from build123d import *

# Parameters (mm, degrees)
CORTAR_EXTRUIR1_DEPTH      = 12.5875
CORTAR_EXTRUIR1_DEPTH_BACK = 12.5875
CORTAR_EXTRUIR2_DEPTH      = 12.5875001
CORTAR_EXTRUIR2_DEPTH_BACK = 12.5875001
CORTAR_EXTRUIR3_DEPTH      = 12.5875001
CORTAR_EXTRUIR3_DEPTH_BACK = 12.5875001


with BuildPart() as part:
    # Croquis1 → Revolución1 (revolve)
    with BuildSketch(Plane.XY):
        Polygon((-61.538063792, 11.5875), (-19.948063792, 11.5875), (-19.948063792, 8.4125), (-17.448063792, 8.4125), (-17.448063792, 2.38125), (0, 2.38125), (0, 1.5875), (-17.448063792, 1.5875), (-21.538063792, 1.5875), (-21.538063792, 10), (-61.538063792, 10), align=None)
    revolve(axis=Axis((0, 0, 0), (-1, 0, 0)))

    # Croquis2 → Cortar-Extruir1 (cut, two sides)
    with BuildSketch(Plane.XY) as cortar_extruir1_sk:
        with BuildLine():
            Line((-40, 2.5), (-30, 2.5))
            ThreePointArc((-30, 2.5), (-27.5, 0), (-30, -2.5))
            Line((-30, -2.5), (-40, -2.5))
            ThreePointArc((-40, -2.5), (-42.5, 0), (-40, 2.5))
        make_face()
    extrude(amount=CORTAR_EXTRUIR1_DEPTH, mode=Mode.SUBTRACT)
    extrude(cortar_extruir1_sk.sketch, amount=-CORTAR_EXTRUIR1_DEPTH_BACK, mode=Mode.SUBTRACT)

    # Croquis3 → Cortar-Extruir2 (cut, two sides)
    with BuildSketch(Plane(origin=(0, 0, 0), x_dir=(1, 0, 0), z_dir=(0, 1, 0))) as cortar_extruir2_sk:
        with BuildLine():
            Line((-40, 2.5), (-30, 2.5))
            ThreePointArc((-30, 2.5), (-27.5, 0), (-30, -2.5))
            Line((-30, -2.5), (-40, -2.5))
            ThreePointArc((-40, -2.5), (-42.5, 0), (-40, 2.5))
        make_face()
    extrude(amount=CORTAR_EXTRUIR2_DEPTH, mode=Mode.SUBTRACT)
    extrude(cortar_extruir2_sk.sketch, amount=-CORTAR_EXTRUIR2_DEPTH_BACK, mode=Mode.SUBTRACT)

    # Croquis4 → Cortar-Extruir3 (cut, two sides)
    with BuildSketch(Plane.XY) as cortar_extruir3_sk:
        Polygon((0, 2.38125), (-0.839757246, -2.38125), (0, -2.38125), align=None)
    extrude(amount=CORTAR_EXTRUIR3_DEPTH, mode=Mode.SUBTRACT)
    extrude(cortar_extruir3_sk.sketch, amount=-CORTAR_EXTRUIR3_DEPTH_BACK, mode=Mode.SUBTRACT)


solid = part.part
The model under review builds one solid part; all positions refer to its coordinate system, in mm. A direction names the side the tool comes from. Coordinates: 2 decimals unless noted, no trailing zeros. Write each loop counter-clockwise with the first axis right and the second up, starting at its lowest first coordinate (ties: lowest second). Pieces come first, ordered by that corner, then holes. Notation, with made-up numbers: M 73.25,5.25 L 112.25,5.25 A8 ccw 112.25,19.25 Z; hole C -28.5,11 d2. An arc over 180 degrees is marked long. Put each result on its own line as item: value.
1) Add section C-C on y = 0. Give the boundary of the cut face in (x, z).
Computed:
outline: M -61.54,-11.59 L -42.5,-11.59 L -42.5,-10 L -61.54,-10 Z; M -61.54,10 L -42.5,10 L -42.5,11.59 L -61.54,11.59 Z; M -27.5,-11.59 L -19.95,-11.59 L -19.95,-8.41 L -17.45,-8.41 L -17.45,-2.38 L -0.42,-2.38 L -0.42,-1.59 L -21.54,-1.59 L -21.54,-10 L -27.5,-10 Z; M -27.5,10 L -21.54,10 L -21.54,1.59 L -0.42,1.59 L -0.42,2.38 L -17.45,2.38 L -17.45,8.41 L -19.95,8.41 L -19.95,11.59 L -27.5,11.59 Z
2) Add section D-D on x = -5.5. Give the boundary of the cut face in (y, z) (1 decimal), then the cut area to 3 significant figures.
Computed:
outline: C 0,0 d4.8; hole C 0,0 d3.2
area: 9.90 mm2
3) Add section A-A on x = -35.5. Give the boundary of the cut face in (y, z) (1 decimal), then the cut area to 3 significant figures.
Computed:
outline: M -11.3,-2.5 A11.6 ccw -2.5,-11.3 L -2.5,-9.7 A10 cw -9.7,-2.5 Z; M -11.3,2.5 L -9.7,2.5 A10 cw -2.5,9.7 L -2.5,11.3 A11.6 ccw Z; M 2.5,-11.3 A11.6 ccw 11.3,-2.5 L 9.7,-2.5 A10 cw 2.5,-9.7 Z; M 2.5,9.7 A10 cw 9.7,2.5 L 11.3,2.5 A11.6 ccw 2.5,11.3 Z
area: 75.6 mm2
4) Add section B-B on z = -0.75. Give the boundary of the cut face in (x, y).
Computed:
outline: M -61.54,-11.56 L -42.38,-11.56 L -42.38,-9.97 L -61.54,-9.97 Z; M -61.54,9.97 L -42.38,9.97 L -42.38,11.56 L -61.54,11.56 Z; M -27.62,-11.56 L -19.95,-11.56 L -19.95,-8.38 L -17.45,-8.38 L -17.45,-2.26 L -0.82,-2.26 L -0.67,-1.4 L -21.54,-1.4 L -21.54,-9.97 L -27.62,-9.97 Z; M -27.62,9.97 L -21.54,9.97 L -21.54,1.4 L -0.17,1.4 L -0.02,2.26 L -17.45,2.26 L -17.45,8.38 L -19.95,8.38 L -19.95,11.56 L -27.62,11.56 Z
5) For faces 4 (the cylindrical face through (-27.5, -10.6, -0.1)), 5 (the flat face through (-19.948, -6.1, -6.1)), 6 (the cylindrical face through (-42.5, -0.1, 10.6)), 7 (the cylindrical face through (-40.45, 5.35, 10.28)), list the 3-axis set-ups (+Z, -Z, +X, -X, +Y, -Y) from which the entire face can be reached by the end or side of a thin tool; tool diameter is ignored.
Computed:
face 4: +Y, -Y
face 5: +X
face 6: +Z, -Z
face 7: +X, -X
6) Draft analysis for pull direction Z (two halves, no side actions). For faces 1 (the cylindrical face through (-8.6, -1.89, 1.45)), 2 (the flat face through (-35, 2.5, -10)), 3 (the flat face through (-35, 10, -2.5)), state which applies: released by +Z, released by -Z, zero draft, split by the parting line, or undercut.
Computed:
face 1: split by the parting line
face 2: zero draft
face 3: undercut
7) Wall thickness on probe 1 along Z at (x, y) = (-46.5, 0); probe 2 along Z at (x, y) = (-9.25, 0): over which ranges is each line inside the solid? List them lowest first. Write a range as [from, to].
Computed:
probe 1: z = [-11.59, -10], [10, 11.59]
probe 2: z = [-2.38, -1.59], [1.59, 2.38]
8) Clearance check with flat-ended pins moving along their axes: pin 1 Ø8 at (y, z) = (-4.5, 0) entering from +X; pin 2 Ø0.8 at (x, y) = (-33, 11) entering from -Z; pin 3 Ø0.5 at (x, y) = (-36, -10.5) entering from -Z. State where each tip first meets the part, or that it passes through.
Computed:
pin 1: stops at x = -0.55
pin 2: stops at z = -4.68
pin 3: stops at z = -5.4
